Verification items for the finished model (mm, model axes). A direction names the side the tool comes from. Coordinates: 2 decimals unless noted, no trailing zeros. Loops run counter-clockwise (first coordinate to the right, second up) from the corner with the lowest first, then second, coordinate; pieces in that order, holes last. Notation, with made-up numbers: (25.25, -4) -> (33.25, -4) arc R11 ccw to (33.25, 4) -> close; hole circle Ø11 at (12.5, -20). An arc over 180 degrees is marked (long way). Answer as a JSON object with one key per item and string values. Group by question number.
Q1. Cross-section at D-D on x = -1.25. Record the boundary of the cut face in (y, z).
Q2. Cross-section at B-B on x = -5. Record the boundary of the cut face in (y, z) (3 decimals), and give its area (3 significant figures).
Q3. Set-up check for faces 1 (the flat face through (-2.7, 10, -2.7)), 2 (the flat face through (-3.8, 7, -3.8)): record each of +Z, -Z, +X, -X, +Y, -Y from which the full face is reachable in a straight line by a thin tool's end or side.
Q4. Gauge pin test, flat ends, axial feed: pin 1 Ø1.7 at (x, z) = (-6.5, -5) entering from +Y; pin 2 Ø2.5 at (x, z) = (-5, -5) entering from +Y. Record the tip position at first contact, or that the pin passes through.
Q5. Release check for a two-part mould opening along X. For faces 3 (the cylindrical face through (-3.48, 8.52, -7.38)), 4 (the cylindrical face through (-1, 6, -5)), 5 (the flat face through (-2, 5, -5)), 6 (the flat face through (-10, 5, -5)) record: released by +X, released by -X, zero draft, split by the parting line, or undercut.
Q6. Cross-section at C-C on y = 5. Record the boundary of the cut face in (x, z) (3 decimals).
Q7. Scan lines: L1, parallel to X at y = 2.75, z = -5 (3 decimals); L2, parallel to Z at x = -5, y = 9.35 (3 decimals). Record each from-to range of solid material in increasing order.
Q8. Cross-section at A-A on z = -5. Record the boundary of the cut face in (x, y) (3 decimals), and give its area (3 significant figures).
Autodesk Inventor part; units mm, degrees
ref_plane "YZ Plane" through (0, 0, 0) normal (1, 0, 0) x (0, 1, 0)
ref_plane "XZ Plane" through (0, 0, 0) normal (0, 1, 0) x (-1, 0, 0)
ref_plane "XY Plane" through (0, 0, 0) normal (0, 0, 1) x (1, 0, 0)
sketch "Sketch1" plane through (0, 0, 0) normal (0, 1, 0) x (-1, 0, 0)
  line L0 (10, 0) -> (0, 0)
  line L1 (0, 0) -> (0, -10)
  line L2 (0, -10) -> (10, -10)
  line L3 (10, -10) -> (10, 0)
  dimension "d0" = 10
  dimension "d1" = 10
extrude "Extrusion1" add sketch "Sketch1" along normal blind 10
sketch "Sketch2" plane through (0, 10, 0) normal (0, 1, 0) x (1, 0, 0)
  line L0 (-10, 0) -> (0, 0) construction
  line L1 (0, 0) -> (0, 10) construction
  line L2 (0, 10) -> (-10, 10) construction
  line L3 (-10, 10) -> (-10, 0) construction
  circle A0 centre (-5, 5) radius 2.825
  dimension "d4" = 5.65
extrude "Extrusion2" cut sketch "Sketch2" against normal blind 3
sketch "Sketch3" plane through (-5, 7, -5) normal (0, 1, 0) x (1, 0, 0)
  circle A0 centre (0, 0) radius 1.425
  point P0 (5, -5)
  dimension "d7" = 2.85
extrude "Extrusion3" cut sketch "Sketch3" against normal through all
sketch "Sketch4" plane through (0, 0, 0) normal (1, 0, 0) x (0, 0, -1)
  line L0 (0, 0) -> (10, 0) construction
  line L1 (10, 0) -> (10, 10) construction
  line L2 (0, 10) -> (10, 10) construction
  line L3 (0, 0) -> (0, 10) construction
  circle A0 centre (5, 5) radius 1 construction
  circle A1 centre (5, 5) radius 1
  dimension "d10" = 2
extrude "Extrusion4" cut sketch "Sketch4" against normal blind 2
properties part number "cubo_calibracion_tornillo_1cm"
Computed values:
{
 "1": {"outline": "(0, -10) -> (10, -10) -> (10, 0) -> (0, 0) -> close; hole circle Ø2 at (5, -5)"},
 "2": {"outline": "(0, -10) -> (10, -10) -> (10, -7.825) -> (7, -7.825) -> (7, -6.425) -> (0, -6.425) -> close; (0, -3.575) -> (7, -3.575) -> (7, -2.175) -> (10, -2.175) -> (10, 0) -> (0, 0) -> close", "area": "63.1 mm²"},
 "3": {"face 1": "+Z, -Z, +X, -X, +Y", "face 2": "+Y"},
 "4": {"pin 1": "stops at y = 7", "pin 2": "passes through"},
 "5": {"face 3": "undercut", "face 4": "zero draft", "face 5": "released by +X", "face 6": "released by -X"},
 "6": {"outline": "(-10, -10) -> (0, -10) -> (0, -6) -> (-2, -6) -> (-2, -4) -> (0, -4) -> (0, 0) -> (-10, 0) -> close; hole circle Ø2.85 at (-5, -5)"},
 "7": {"L1": "x = -10 to -6.425, -3.575 to 0", "L2": "z = -10 to -7.825, -2.175 to 0"},
 "8": {"outline": "(-10, 0) -> (-6.425, 0) -> (-6.425, 7) -> (-7.825, 7) -> (-7.825, 10) -> (-10, 10) -> close; (-3.575, 0) -> (0, 0) -> (0, 4) -> (-2, 4) -> (-2, 6) -> (0, 6) -> (0, 10) -> (-2.175, 10) -> (-2.175, 7) -> (-3.575, 7) -> close", "area": "59.1 mm²"}
}
